Autodesk Fusion 360 part; units mm, degrees
sketch "Sketch1" plane through (0, 0, 0) normal (0, 0, 1) x (1, 0, 0)
  circle A0 centre (0, 0) radius 6
  circle A1 centre (0, 0) radius 2.5
  dimension "d1" = 12
  dimension "d2" = 5
extrude "Extrude1" add sketch "Sketch1" along normal blind 6.5 makes body 1
sketch "Sketch2" plane through (0, 0, 6.5) normal (0, 0, 1) x (1, 0, 0)
  circle A0 centre (0, 0) radius 2.5
  circle A1 centre (0, 0) radius 6
  circle A2 centre (0, 0) radius 7.95
  dimension "d5" = 15.9
extrude "Extrude2" add sketch "Sketch2" along normal blind 1 contours A1 | A2 bodies 1
sketch "Sketch3" plane through (0, 0, 7.5) normal (0, 0, 1) x (1, 0, 0)
  circle A0 centre (0, 0) radius 2.5
  circle A1 centre (0, 0) radius 7.95
  circle A2 centre (0, 0) radius 4.75
  circle A3 centre (0, 0) radius 4.55
  circle A4 centre (0, 0) radius 4.05
  circle A5 centre (0, 0) radius 3
  dimension "d8" = 3.2
  dimension "d9" = 0.2
  dimension "d10" = 0.5
  dimension "d11" = 0.5
extrude "Extrude3" cut sketch "Sketch3" against normal blind 0.2 contours A2 bodies 1
chamfer "Chamfer1" distance 0.2 angle 45 1 edges at (-4.4286, 1.7177, 7.3) on bodies 1
extrude "Extrude4" cut sketch "Sketch3" against normal blind 0.2 contours A4 bodies 1
split "Split1" by plane through (0, 0, 6.5) normal (0, 0, -1) bodies 1 makes body 2 at (5.9925, -0.2991, 2.1667)
ref_plane "WorkPlane1" through (0, 0, 3.25) normal (0, 0, -1) x (-1, 0, 0)
mirror "Mirror1" about plane through (0, 0, 3.25) normal (0, 0, -1) of bodies 1 makes body 3
combine "Combine1" operation add target body 1 tool bodies 2 3
chamfer "Chamfer2" distance 0.5 angle 45 2 edges at (-7.412, -2.8748, 7.5) (-7.412, -2.8748, -1) on bodies 1
equation "d17 = ( -6.5 / 2 ) * 1 mm"
Part model, mm, in its own coordinate system. A direction names the side the tool comes from. Coordinates: 2 decimals unless noted, no trailing zeros. Order: outer loops, then holes, each group sorted by start corner. A loop starts at its lowest first (then second) coordinate and runs counter-clockwise, first axis right, second up. Notation, with made-up numbers: (5.25, 69.25) -> (50.25, 69.25) arc R21 cw to (50.25, 92.25) -> close; hole circle Ø7 at (-8, 24.25). An arc over 180 degrees is marked (long way). Put each result on its own line as item: value. Start each with the question number.
(1) Mould opens along Y. For faces 1 (the face through (0, -5, 7.5)), 2 (the face through (-0.54, -2.44, 3.31)), 3 (the face through (-1.72, -7.76, -0.25)) say: pulls with the +Y half, pulls with the -Y half, needs draft (parallel to the pull), parting line crosses it, or undercut.
(2) Probe line 1 along Z through (x, y) = (-2.25, 6.5); line 2 along Z through (x, y) = (3, 2.5); line 3 along Y through (x, z) = (0, 7.45). List the from-to ranges inside material, lowest first. Write a range as [from, to].
(3) Which spindle directions (+Z, -Z, +X, -X, +Y, -Y) get a long thin tool onto all of the face, cutting with end or side? Do faces 4 (the face through (3, -3, -1)), 5 (the face through (2, 6, 0)). Say none if no direction does.
(4) Pin check, flat tips, straight feed: pin 1 Ø2 at (y, z) = (1.5, 5) entering from +X; pin 2 Ø2 at (x, z) = (-1, 1.5) entering from -Y; pin 3 Ø1.5 at (y, z) = (-2, 5.5) entering from +X. Stop position of each tip, or through.
(5) Band-saw the part on A-A (z = 6). Give the cut face in (x, y), then the cut area to 3 significant figures.
Determined:
1. face 1: needs draft
1. face 2: undercut
1. face 3: parting line crosses it
2. line 1: z = [-1, 0], [6.5, 7.5]
2. line 2: z = [-0.8, 7.3]
2. line 3: y = [-7.5, -4.7], [-4.55, -4.05], [-3, -2.5], [2.5, 3], [4.05, 4.55], [4.7, 7.5]
3. face 4: -Z, +X, -X, +Y, -Y
3. face 5: none
4. pin 1: stops at x = 5.98
4. pin 2: stops at y = -6
4. pin 3: stops at x = 5.87
5. outline: circle Ø12 at (0, 0); hole circle Ø5 at (0, 0)
5. area: 93.5 mm²
